Here's how the part is built. I have some questions about the finished solid (model axes, mm). Face numbers are marked on the shaded views. A direction names the side the tool comes from. Coordinates: 2 decimals unless noted, no trailing zeros. Write each loop counter-clockwise with the first axis right and the second up, starting at its lowest first coordinate (ties: lowest second). Pieces come first, ordered by that corner, then holes.
Item 1: If we section it at C-C (x = 5): Please give me the cut outline in (y, z), then the cut area to 3 significant figures.
Item 2: If we section it at D-D (y = -4.25): Please give me the cut outline in (x, z).
Item 3: I'm going to push flat-ended pins straight in: pin 1 Ø2 at (x, z) = (23, 7.5) entering from +Y; pin 2 Ø1.8 at (y, z) = (2.5, -10) entering from -X; pin 3 Ø9.5 at (x, z) = (-42, 1.5) entering from -Y. Where does each tip first touch, or does it pass through?
Item 4: For the marked faces 1, 2, 3 and 4, which set-ups out of +Z, -Z, +X, -X, +Y, -Y let a thin tool reach every point of the face, with its end or its side?
Item 5: If we section it at A-A (y = 2): Please give me the cut outline in (x, z), then the cut area to 3 significant figures.
Item 6: If we section it at B-B (z = 3): Please give me the cut outline in (x, y).
Item 7: If I drill on line 1 (Y direction, x = -3.5, z = -9.5); line 2 (X direction, y = -16, z = -5); line 3 (Z direction, x = -28, y = -9.25), over which ranges is the centre line in solid material (lowest first)?
from build123d import *

# Parameters (mm, degrees)
SKETCH1_W           = 65
SKETCH1_H           = 28
BOSS_EXTRUDE1_DEPTH = 21
SKETCH3_W           = 4
SKETCH3_H           = 8
BOSS_EXTRUDE2_DEPTH = 6
SKETCH3_3_W         = 8
SKETCH3_3_H         = 8
BOSS_EXTRUDE3_DEPTH = 6
SKETCH4_W           = 8
SKETCH4_H           = 3
BOSS_EXTRUDE4_DEPTH = 20
SKETCH5_W           = 8
SKETCH5_H           = 6
BOSS_EXTRUDE5_DEPTH = 5


with BuildPart() as part:
    # Sketch1 → Boss-Extrude1 (new body)
    with BuildSketch(Plane(origin=(0, 0, 0), x_dir=(1, 0, 0), z_dir=(0, 1, 0))):
        Rectangle(SKETCH1_W, SKETCH1_H)
    extrude(amount=-BOSS_EXTRUDE1_DEPTH)

    # Sketch3 → Boss-Extrude2 (add)
    with BuildSketch(Plane(origin=(0, 0, 0), x_dir=(1, 0, 0), z_dir=(0, 1, 0))):
        with Locations((-30.5, 0)):
            Rectangle(SKETCH3_W, SKETCH3_H)
    extrude(amount=BOSS_EXTRUDE2_DEPTH)

    # Sketch3_3 → Boss-Extrude3 (add)
    with BuildSketch(Plane(origin=(0, 0, 0), x_dir=(1, 0, 0), z_dir=(0, 1, 0))):
        with Locations((-21.5, 10)):
            Rectangle(SKETCH3_3_W, SKETCH3_3_H)
    extrude(amount=BOSS_EXTRUDE3_DEPTH)

    # Sketch4 → Boss-Extrude4 (add)
    with BuildSketch(Plane.ZY.offset(32.5)):
        Polygon((-4, 6), (4, 6), (4, 3), (4, 0), (6, 0), (6, 7.5), (-6, 7.5), (-6, 0), (-4, 0), (-4, 3), align=None)
        with Locations((0, 4.5)):
            Rectangle(SKETCH4_W, SKETCH4_H)
        Polygon((4, 0), (4, 3), (-4, 3), (-4, 0), (-6, 0), (-6, -1.5), (6, -1.5), (6, 0), align=None)
    extrude(amount=BOSS_EXTRUDE4_DEPTH)

    # Sketch5 → Boss-Extrude5 (add)
    with BuildSketch(Plane(origin=(0, 0, -14), x_dir=(-1, 0, 0), z_dir=(0, 0, -1))):
        with Locations((21.5, 3)):
            Rectangle(SKETCH5_W, SKETCH5_H)
    extrude(amount=BOSS_EXTRUDE5_DEPTH)


solid = part.part
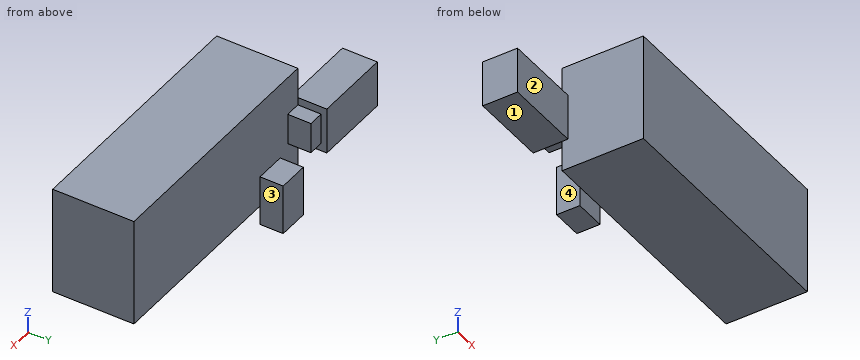
Answer list:
1. outline: (-21, -14) - (0, -14) - (0, 14) - (-21, 14) - close
1. area: 588 mm2
2. outline: (-32.5, -14) - (32.5, -14) - (32.5, 14) - (-32.5, 14) - close
3. pin 1: stops at y = 0
3. pin 2: stops at x = -25.5
3. pin 3: stops at y = -1.5
4. face 1: -Z, -X, +Y, -Y
4. face 2: +Z, -Z, -X, -Y
4. face 3: +Z, -Z, +X, +Y
4. face 4: +Z, -Z, -X, +Y
5. outline: (-52.5, -6) - (-32.5, -6) - (-32.5, -4) - (-28.5, -4) - (-28.5, 4) - (-32.5, 4) - (-32.5, 6) - (-52.5, 6) - close; (-25.5, -19) - (-17.5, -19) - (-17.5, -6) - (-25.5, -6) - close
5. area: 376 mm2
6. outline: (-52.5, -1.5) - (-32.5, -1.5) - (-32.5, -21) - (32.5, -21) - (32.5, 0) - (-28.5, 0) - (-28.5, 6) - (-32.5, 6) - (-32.5, 7.5) - (-52.5, 7.5) - close
7. line 1: y = -21 to 0
7. line 2: x = -32.5 to 32.5
7. line 3: z = -14 to 14
